Answer from the drawing. Dimensions are ordinates in mm from the lowest x, y and z of the part. Round coordinates to 2 decimals unless told otherwise and drop trailing zeros. Order: outer loops, then holes, each group sorted by start corner. A loop starts at its lowest first (then second) coordinate and runs counter-clockwise, first axis right, second up. Notation, with made-up numbers: (67.25, 80.5) -> (120.25, 80.5) arc R18 cw to (120.25, 99.5) -> close; hole circle Ø11 at (66, 1). An arc over 180 degrees is marked (long way). Use a Markdown table: item, result. Add a question column.
Item 1: Find the intervals of material crossed by L1, parallel to X at y = 6, z = 0.5; L2, parallel to X at y = 4.5, z = 7.75 (1 decimal); L3, parallel to Y at x = 12, z = 4 (1 decimal), in increasing order. Write a range as [from, to].
Item 2: A cutting plane is placed at B-B, the plane z = 1.25. Determine the outline of the cut face in (x, y) (1 decimal), plus the area to 3 significant figures.
Item 3: A cutting plane is placed at C-C, the plane x = 36. Determine the outline of the cut face in (y, z), plus the area to 3 significant figures.
Item 4: A cutting plane is placed at A-A, the plane y = 4.25. Determine the outline of the cut face in (x, z) (1 decimal).
Item 5: A cutting plane is placed at D-D, the plane z = 7.75. Determine the outline of the cut face in (x, y).
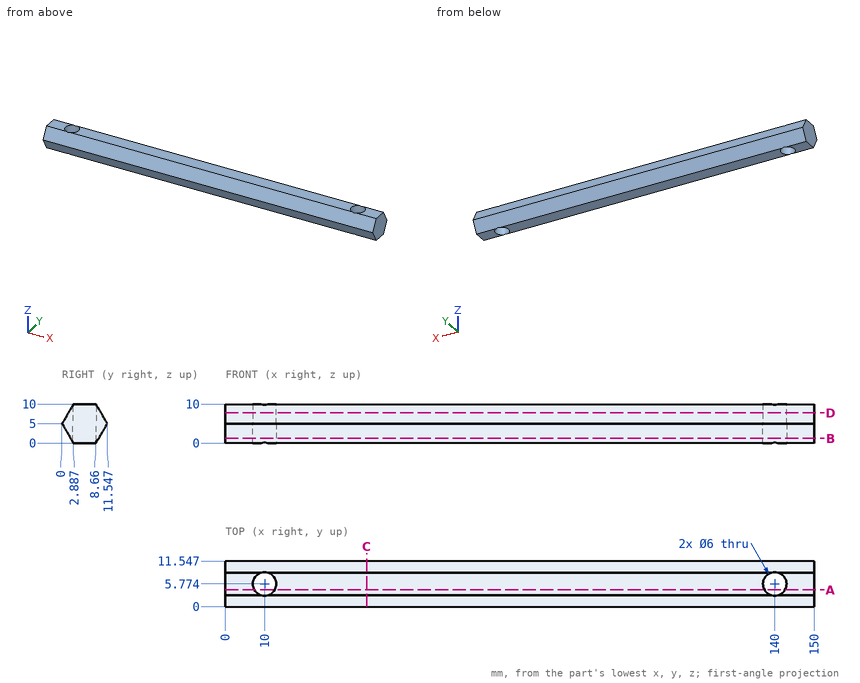
Reported:
| question | item | result |
|---|---|---|
| 1 | L1 | [0, 7.01], [12.99, 137.01], [142.99, 150] |
| 1 | L2 | [0, 7.3], [12.7, 137.3], [142.7, 150] |
| 1 | L3 | [0.6, 3.5], [8, 11] |
| 2 | outline | (0, 2.2) -> (150, 2.2) -> (150, 9.4) -> (0, 9.4) -> close; hole circle Ø6 at (10, 5.8); hole circle Ø6 at (140, 5.8) |
| 2 | area | 1,030 mm² |
| 3 | outline | (0, 5) -> (2.89, 0) -> (8.66, 0) -> (11.55, 5) -> (8.66, 10) -> (2.89, 10) -> close |
| 3 | area | 86.6 mm² |
| 4 | outline | (0, 0) -> (7.4, 0) -> (7.4, 10) -> (0, 10) -> close; (12.6, 0) -> (137.4, 0) -> (137.4, 10) -> (12.6, 10) -> close; (142.6, 0) -> (150, 0) -> (150, 10) -> (142.6, 10) -> close |
| 5 | outline | (0, 1.59) -> (150, 1.59) -> (150, 9.96) -> (0, 9.96) -> close; hole circle Ø6 at (10, 5.77); hole circle Ø6 at (140, 5.77) |
